Autodesk Inventor part; units mm, degrees
ref_plane "YZ Plane" through (0, 0, 0) normal (1, 0, 0) x (0, 1, 0)
ref_plane "XZ Plane" through (0, 0, 0) normal (0, 1, 0) x (-1, 0, 0)
ref_plane "XY Plane" through (0, 0, 0) normal (0, 0, 1) x (1, 0, 0)
sketch "Sketch1" plane through (0, 0, 0) normal (0, 0, 1) x (1, 0, 0)
  circle A0 centre (0, 0) radius 14.5
  dimension "d0" = 29
extrude "Extrusion1" add sketch "Sketch1" along normal blind 1.5
sketch "Sketch2" plane through (0, 0, 0) normal (0, 0, -1) x (-1, 0, 0)
  circle A0 centre (0, 0) radius 14.5
  circle A1 centre (0, 0) radius 13
  dimension "d3" = 26
extrude "Extrusion2" add sketch "Sketch2" along normal blind 7 contours A1
sketch "Sketch3" plane through (0, 0, -7) normal (0, 0, -1) x (-1, 0, 0)
  circle A0 centre (0, 0) radius 13
  circle A1 centre (0, 0) radius 14.5
  dimension "d6" = 29
extrude "Extrusion3" add sketch "Sketch3" along normal blind 1.5 contours A0 | A1
sketch "Sketch4" plane through (0, 0, 1.5) normal (0, 0, 1) x (1, 0, 0)
  circle A0 centre (0, 0) radius 14.5
hole "Hole1" at (0, 0, 1.5) direction (0, 0, -1) diameter 4.134 end through all
properties part number "20 - Piston" material "Steel AISI 1020 107 HR"
The model under review builds one solid part; all positions refer to its coordinate system, in mm. A direction names the side the tool comes from. Give positions to 0.01 mm unless a question says otherwise; leave off trailing zeros. Loops run counter-clockwise (first coordinate to the right, second up) from the corner with the lowest first, then second, coordinate; pieces in that order, holes last. Notation, with made-up numbers: (21, 41) -> (72, 41) arc R8 cw to (72, 55) -> close; hole circle Ø2 at (27.5, -32.75). An arc over 180 degrees is marked (long way). Answer as a JSON object with one key per item and string values. Group by question number.
Q1. Draft analysis for pull direction Z (two halves, no side actions). For faces 1 (the cylindrical face through (1.26, 1.64, -3.57)), 2 (the flat face through (-9, 10, 0)), 3 (the flat face through (3, 0, 1.5)), state which applies: pulls with the +Z half, pulls with the -Z half, needs draft (parallel to the pull), parting line crosses it, or undercut.
Q2. Take a section at D-D (z = -7.5). Write out the cut boundary in (x, y), plus the area to 3 significant figures.
Q3. Take a section at A-A (y = 0). Write out the cut boundary in (x, z).
Q4. Take a section at C-C (y = 10.5). Write out the cut boundary in (x, z).
Q5. Tool access review of faces 4 (the cylindrical face through (10.316, 7.91, -3.451)), 5 (the flat face through (-3, 0, -8.5)): name each direction out of +Z, -Z, +X, -X, +Y, -Y from which nothing blocks a thin tool from reaching the whole face with its end or side.
Q6. Wall thickness on line 1 along Z through (x, y) = (-8.25, 11.25); line 2 along Y through (x, z) = (0, -0.75); line 3 along Y through (x, z) = (2.75, -5.5): over which ranges is each line inside the solid? List them lowest first.
Q7. Insertion check: pin 1 (4 mm diameter, centred on x = 6.5, z = -6, fed in from -Y); pin 2 (1 mm diameter, centred on y = 4.5, z = -4.5, fed in from +X); pin 3 (3 mm diameter, centred on x = 8.5, z = -4.5, fed in from -Y). Each pin has a flat end and moves straight along its axis. Give the tip position at first contact, or say it passes through.
Answer below:
{
 "1": {"face 1": "needs draft", "face 2": "undercut", "face 3": "pulls with the +Z half"},
 "2": {"outline": "circle Ø29 at (0, 0); hole circle Ø4.13 at (0, 0)", "area": "647 mm2"},
 "3": {"outline": "(-14.5, -8.5) -> (-2.07, -8.5) -> (-2.07, 1.5) -> (-14.5, 1.5) -> (-14.5, 0) -> (-13, 0) -> (-13, -7) -> (-14.5, -7) -> close; (2.07, -8.5) -> (14.5, -8.5) -> (14.5, -7) -> (13, -7) -> (13, 0) -> (14.5, 0) -> (14.5, 1.5) -> (2.07, 1.5) -> close"},
 "4": {"outline": "(-10, -8.5) -> (10, -8.5) -> (10, -7) -> (7.66, -7) -> (7.66, 0) -> (10, 0) -> (10, 1.5) -> (-10, 1.5) -> (-10, 0) -> (-7.66, 0) -> (-7.66, -7) -> (-10, -7) -> close"},
 "5": {"face 4": "none", "face 5": "-Z, +X, -X, +Y, -Y"},
 "6": {"line 1": "z = -8.5 to -7, 0 to 1.5", "line 2": "y = -13 to -2.07, 2.07 to 13", "line 3": "y = -12.71 to 12.71"},
 "7": {"pin 1": "stops at y = -13.69", "pin 2": "stops at x = 12.37", "pin 3": "stops at y = -10.95"}
}
